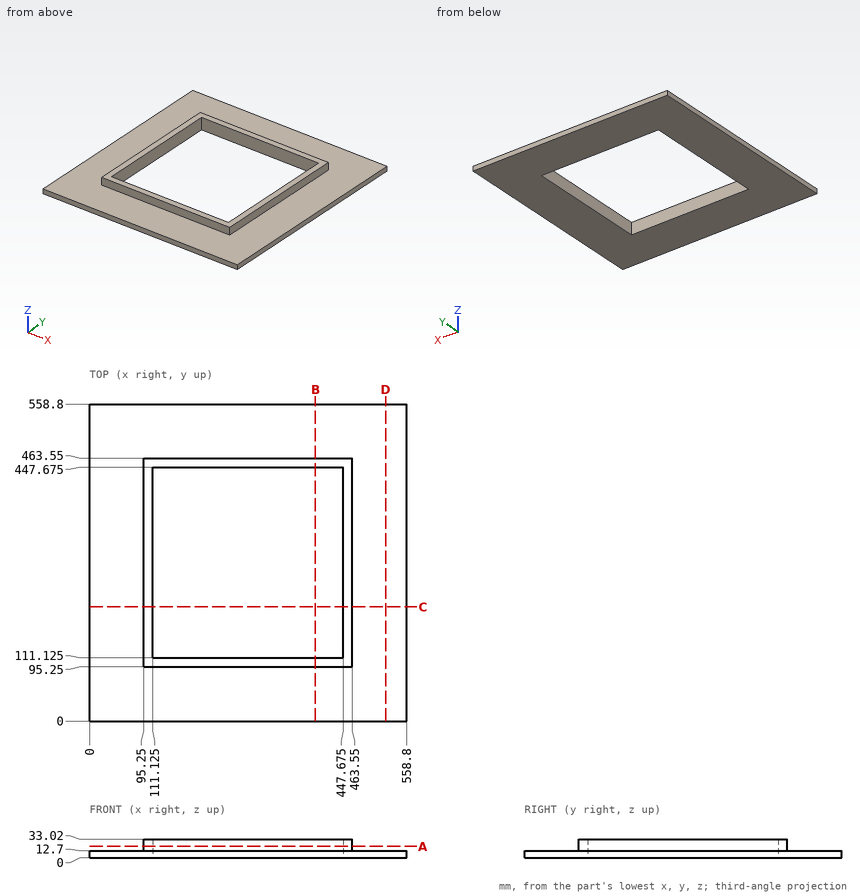
Verification items for this drawing (mm, ordinates from the low corner). Coordinates: 2 decimals unless noted, no trailing zeros. Write each loop counter-clockwise with the first axis right and the second up, starting at its lowest first coordinate (ties: lowest second). Pieces come first, ordered by that corner, then holes. Notation, with made-up numbers: M -31.5,15.25 L -20.5,15.25 A12 ccw -20.5,24.25 Z; hole C 7,55.25 d7. An arc over 180 degrees is marked long. Use CSV: the item, a comma, the result in double quotes.
Q1. Thickness scan on line 1 along X through (y, z) = (225, 22.5) (3 decimals); line 2 along Y through (x, z) = (289.5, 8) (3 decimals). Record the ranges inside material, lowest first. Write a range as [from, to].
Computed values:
line 1,"[95.25, 111.125], [447.675, 463.55]"
line 2,"[0, 111.125], [447.675, 558.8]"
Q2. Section check B-B, the plane x = 398. Enter the section's corners in (y, z) (3 decimals).
Computed values:
outline,"M 0,0 L 111.125,0 L 111.125,33.02 L 95.25,33.02 L 95.25,12.7 L 0,12.7 Z; M 447.675,0 L 558.8,0 L 558.8,12.7 L 463.55,12.7 L 463.55,33.02 L 447.675,33.02 Z"
Q3. Section check D-D, the plane x = 522. Enter the section's corners in (y, z).
Computed values:
outline,"M 0,0 L 558.8,0 L 558.8,12.7 L 0,12.7 Z"
Q4. Section check A-A, the plane z = 20. Enter the section's corners in (x, y) (3 decimals), and give its area (3 significant figures).
Computed values:
outline,"M 95.25,95.25 L 463.55,95.25 L 463.55,463.55 L 95.25,463.55 Z; hole M 111.125,111.125 L 447.675,111.125 L 447.675,447.675 L 111.125,447.675 Z"
area,"22,400 mm²"
Q5. Go/stop test with flat-tipped pins: P1, Ø10, axis at y = 271.5, z = 18, coming from the -X side; P2, Ø10, axis at y = 180, z = 22.5, coming from the +X side; P3, Ø6, axis at x = 195.5, z = 26.5, coming from the +Y side. Record where each tip stops, or that it passes through.
Computed values:
P1,"x = 95.25"
P2,"x = 463.55"
P3,"y = 463.55"
